Read the model definition and answer for the solid it produces. Units are mm, in the model's axes. A direction names the side the tool comes from. Coordinates: 2 decimals unless noted, no trailing zeros. Order: outer loops, then holes, each group sorted by start corner. A loop starts at its lowest first (then second) coordinate and runs counter-clockwise, first axis right, second up. Notation, with made-up numbers: (-5, 12.25) - (19, 12.25) arc R10 cw to (19, 17.25) - close; hole circle Ø11 at (77.5, 45). An arc over 180 degrees is marked (long way). Write item = value, one per line.
from build123d import *

# Parameters (mm, degrees)
F0_W     = 30
F0_H     = 50
F1_DEPTH = 7
F2_R     = 4.5
F3_DEPTH = 5
F4_R     = 1.5
F5_DEPTH = 7.001
F7_DEPTH = 7
F8_R     = 1.25
F9_DEPTH = 30.001
F10_SIZE = 1


with BuildPart() as f1:
    # F0 (on Top) → F1 (new body)
    with BuildSketch(Plane.XY):
        with Locations((2.6609585285, -2.2089038044)):
            Rectangle(F0_W, F0_H)
    extrude(amount=F1_DEPTH)

    # F2 (on face) → F3 (cut)
    with BuildSketch(Plane.XY.offset(7)):
        with Locations((2.6609585285, -18.7089038044)):
            Circle(F2_R)
    extrude(amount=-F3_DEPTH, mode=Mode.SUBTRACT)

    # F4 (on face) → F5 (cut, through all)
    with BuildSketch(Plane.XY.offset(7)):
        with Locations((9.3609585285, -8.7089038044)):
            Circle(F4_R)
        with Locations((-4.0390414715, -8.7089038044)):
            Circle(F4_R)
    extrude(amount=-F5_DEPTH, mode=Mode.SUBTRACT)

    # F6 (on face) → F7 (join)
    with BuildSketch(Plane(origin=(0, 0, 0), x_dir=(1, 0, 0), z_dir=(0, 0, -1))):
        Polygon((-9.8390414715, 27.2089038044), (-12.3390414715, 27.2089038044), (-12.3390414715, -22.7910961956), (-9.8390414715, -22.7910961956), (-9.8390414715, -19.8687557131), (-9.8390414715, -19.1495772451), align=None)
        Polygon((17.6609585285, 27.2089038044), (15.1609585285, 27.2089038044), (15.1609585285, -19.1495772451), (15.1609585285, -19.8687557131), (15.1609585285, -22.7910961956), (17.6609585285, -22.7910961956), align=None)
    extrude(amount=F7_DEPTH)

    # F8 (on face) → F9 (cut, through all)
    with BuildSketch(Plane(origin=(-12.3390414715, 0, 0), x_dir=(0, -1, 0), z_dir=(-1, 0, 0))):
        with BuildLine():
            ThreePointArc((-15.7910961956, -7), (-17.3563437798, -6.6304951685), (-18.5910961956, -5.6))
            Line((-18.5910961956, -5.6), (-22.7910961956, 0))
            Line((-22.7910961956, 0), (-22.7910961956, -7))
            Line((-22.7910961956, -7), (-15.7910961956, -7))
        make_face()
        with BuildLine():
            ThreePointArc((15.9661451837, -6.5268965517), (15.1188109615, -6.8796551548), (14.2089038044, -7))
            Line((14.2089038044, -7), (27.2089038044, -7))
            Line((27.2089038044, -7), (27.2089038044, 0))
            Line((27.2089038044, 0), (15.9661451837, -6.5268965517))
        make_face()
        with Locations((14.2089038044, -3.5)):
            Circle(F8_R)
        with Locations((-15.7910961956, -3.5)):
            Circle(F8_R)
    extrude(amount=-F9_DEPTH, mode=Mode.SUBTRACT)

    # F10
    f10_edges = [f1.edges().sort_by_distance(p)[0] for p in [
        (-12.339041, 22.791096, 3.5),
        (-12.339041, 20.691096, -2.8),
        (-12.339041, -27.208904, 3.5),
        (17.660959, -27.208904, 3.5),
        (17.660959, -21.587524, -3.263448),
        (17.660959, 22.791096, 3.5),
        (-1.839041, -18.708904, 7),
        (-5.539041, -8.708904, 7),
        (7.860959, -8.708904, 7),
    ]]
    chamfer(f10_edges, length=F10_SIZE)


solid = f1.part
1) Determine the mould class of faces 1 (the face through (-11.83, 0.58, -6.51)), 2 (the face through (3, -27.209, 4)), 3 (the face through (16.393, 14.636, -3.979)) for opening direction Y: pulls with the +Y half, pulls with the -Y half, needs draft (parallel to the pull), parting line crosses it, or undercut.
Returned:
face_1 = needs draft
face_2 = pulls with the -Y half
face_3 = undercut
2) The part is cut by section C-C (x = 13). Determine the outline of the cut face in (y, z).
Returned:
outline = (-27.21, 0) - (22.79, 0) - (22.79, 7) - (-27.21, 7) - close
3) For faces 4 (the face through (3, -19, 2)), 5 (the face through (17.15, 22.3, 3.55)), 6 (the face through (-9.839, -2, -3)), determine the directions among +Z, -Z, +X, -X, +Y, -Y from which every point of the face is accessible in a straight line to the end or side of a thin tool.
Returned:
face_4 = +Z
face_5 = +Z, -Z, +X, +Y
face_6 = -Z, +Y, -Y
4) Straight lines are drawn through the part: line 1 along X through (y, z) = (-8, -2.75); line 2 along Z through (x, y) = (-4, -13.5); line 3 along Z through (x, y) = (3, -23). For each, find the intervals that lie inside material, in ascending order. Write a range as from..to.
Returned:
line_1 = -12.34..-9.84, 15.16..17.66
line_2 = 0..7
line_3 = 0..2
5) The part is cut by section B-B (z = -1.5). Determine the outline of the cut face in (x, y).
Returned:
outline = (-12.34, -22.63) - (-11.34, -24.63) - (-9.84, -24.63) - (-9.84, 21.67) - (-11.34, 21.67) - (-12.34, 20.42) - close; (15.16, -24.63) - (16.66, -24.63) - (17.66, -22.63) - (17.66, 20.42) - (16.66, 21.67) - (15.16, 21.67) - close
6) The part is cut by section A-A (y = 14). Determine the outline of the cut face in (x, z).
Returned:
outline = (-12.34, -6) - (-11.34, -7) - (-9.84, -7) - (-9.84, 0) - (15.16, 0) - (15.16, -7) - (16.66, -7) - (17.66, -6) - (17.66, 7) - (-12.34, 7) - close
7) A flat-ended cylindrical pin translates along its axis: pin 1 Ø5 at (x, y) = (-4.04, -8.71) entering from -Z. Find the tip coordinate at first contact, or state that the pin passes through.
Returned:
pin_1 = 0
